CAD build for the part. Positions are in the model's coordinates, mm. Give positions to 0.01 mm unless a question says otherwise; leave off trailing zeros. Loops run counter-clockwise (first coordinate to the right, second up) from the corner with the lowest first, then second, coordinate; pieces in that order, holes last.
Autodesk Fusion 360 part; units mm, degrees
sketch "Sketch1" plane through (0, 0, 0) normal (0, 1, 0) x (1, 0, 0)
  line L0 (0.6394, 2.8043) -> (0.4754, 3.1598)
  line L1 (322.165, 133.829) -> (322.508, 133.638)
  line L2 (0.4754, 3.1598) -> (0.339, 3.5278)
  line L3 (324.895, 129.374) -> (324.896, 5.0726)
  line L4 (0.2329, 3.9067) -> (0.1557, 4.2912)
  line L5 (0.339, 3.5278) -> (0.2329, 3.9067)
  line L6 (0.831, 2.4612) -> (0.6394, 2.8043)
  line L7 (0.1557, 4.2912) -> (0.1102, 4.6812)
  line L8 (321.809, 0.4548) -> (321.441, 0.3183)
  line L9 (320.678, 0.135) -> (320.288, 0.0896)
  line L10 (1.2912, 1.8259) -> (1.0487, 2.1346)
  line L11 (324.879, 129.767) -> (324.895, 129.374)
  line L12 (324.514, 131.288) -> (324.651, 130.92)
  line L13 (323.698, 132.623) -> (323.941, 132.314)
  line L14 (324.159, 2.4612) -> (323.941, 2.1346)
  line L15 (324.651, 3.5278) -> (324.514, 3.1598)
  line L16 (323.431, 1.5379) -> (323.143, 1.2705)
  line L17 (324.35, 2.8043) -> (324.159, 2.4612)
  line L18 (324.757, 130.542) -> (324.834, 130.157)
  line L19 (324.834, 4.2912) -> (324.757, 3.9067)
  line L20 (322.508, 0.8103) -> (322.165, 0.6187)
  line L21 (324.757, 3.9067) -> (324.651, 3.5278)
  line L22 (323.698, 1.8259) -> (323.431, 1.5379)
  line L23 (322.834, 1.028) -> (322.508, 0.8103)
  line L24 (322.508, 133.638) -> (322.834, 133.42)
  line L25 (320.288, 0.0896) -> (319.896, 0.073)
  line L26 (322.834, 133.42) -> (323.143, 133.178)
  line L27 (321.062, 134.236) -> (321.441, 134.13)
  line L28 (323.143, 133.178) -> (323.431, 132.91)
  line L29 (324.651, 130.92) -> (324.757, 130.542)
  line L30 (3.9274, 0.2122) -> (3.5485, 0.3183)
  line L31 (324.35, 131.644) -> (324.514, 131.288)
  line L32 (320.288, 134.359) -> (320.678, 134.313)
  line L33 (320.678, 134.313) -> (321.062, 134.236)
  line L34 (321.441, 134.13) -> (321.809, 133.993)
  line L35 (323.941, 132.314) -> (324.159, 131.987)
  line L36 (321.062, 0.2122) -> (320.678, 0.135)
  line L37 (323.143, 1.2706) -> (322.834, 1.028)
  line L38 (321.441, 0.3183) -> (321.062, 0.2122)
  line L39 (319.896, 0.073) -> (5.0946, 0.073)
  line L40 (324.514, 3.1598) -> (324.35, 2.8043)
  line L41 (324.896, 5.0726) -> (324.879, 4.6812)
  line L42 (324.834, 130.157) -> (324.879, 129.767)
  line L43 (5.0946, 0.073) -> (4.7019, 0.0896)
  line L44 (324.879, 4.6812) -> (324.834, 4.2912)
  line L45 (321.809, 133.993) -> (322.165, 133.829)
  line L46 (3.1805, 0.4548) -> (2.825, 0.6187)
  line L47 (319.896, 134.374) -> (320.288, 134.359)
  line L48 (4.3119, 0.135) -> (3.9274, 0.2122)
  line L49 (2.1553, 1.028) -> (1.8466, 1.2706)
  line L50 (2.825, 0.6187) -> (2.4819, 0.8103)
  line L51 (2.4819, 0.8103) -> (2.1553, 1.028)
  line L52 (324.159, 131.987) -> (324.35, 131.644)
  line L53 (322.165, 0.6187) -> (321.809, 0.4548)
  line L54 (4.7019, 0.0896) -> (4.3119, 0.135)
  line L55 (3.5485, 0.3183) -> (3.1805, 0.4548)
  line L56 (323.941, 2.1346) -> (323.698, 1.8259)
  line L57 (323.431, 132.91) -> (323.698, 132.623)
  line L58 (3.1805, 133.993) -> (3.5485, 134.13)
  line L59 (1.8466, 133.178) -> (2.1553, 133.42)
  line L60 (4.3119, 134.313) -> (4.7019, 134.359)
  line L61 (4.7019, 134.359) -> (5.0946, 134.375)
  line L62 (5.0946, 134.375) -> (319.896, 134.374)
  line L63 (3.5485, 134.13) -> (3.9274, 134.236)
  line L64 (1.5586, 1.5379) -> (1.2912, 1.8259)
  line L65 (0.6394, 131.644) -> (0.831, 131.987)
  line L66 (0.4754, 131.288) -> (0.6394, 131.644)
  line L67 (0.1102, 129.767) -> (0.1557, 130.157)
  line L68 (2.1553, 133.42) -> (2.4819, 133.638)
  line L69 (1.8466, 1.2706) -> (1.5586, 1.5379)
  line L70 (0.1102, 4.6812) -> (0.0937, 5.0739)
  line L71 (314.895, 124.375) -> (314.895, 10.0748)
  line L72 (10.0941, 124.375) -> (314.895, 124.375)
  line L73 (3.9274, 134.236) -> (4.3119, 134.313)
  line L74 (0.831, 131.987) -> (1.0487, 132.314)
  line L75 (1.0487, 132.314) -> (1.2912, 132.623)
  line L76 (314.895, 10.0748) -> (10.0941, 10.0748)
  line L77 (0.2329, 130.542) -> (0.339, 130.92)
  line L78 (0.339, 130.92) -> (0.4754, 131.288)
  line L79 (0.0937, 5.0739) -> (0.0951, 129.374)
  line L80 (1.2912, 132.623) -> (1.5586, 132.91)
  line L81 (0.1557, 130.157) -> (0.2329, 130.542)
  line L82 (2.825, 133.829) -> (3.1805, 133.993)
  line L83 (0.0951, 129.374) -> (0.1102, 129.767)
  line L84 (10.0941, 10.0748) -> (10.0941, 124.375)
  line L85 (1.5586, 132.91) -> (1.8466, 133.178)
  line L86 (2.4819, 133.638) -> (2.825, 133.829)
  line L87 (1.0487, 2.1346) -> (0.831, 2.4612)
extrude "Extrude1" add sketch "Sketch1" along normal blind 3
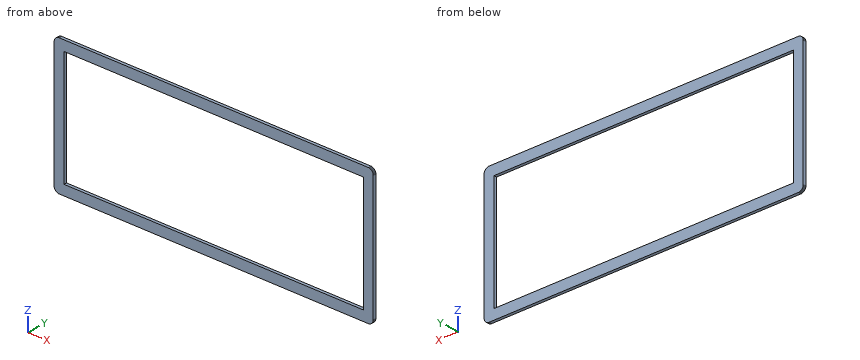
1. Saw through at A-A, the plane x = 276. List the corners of the cut face in (y, z) (3 decimals).
Responses:
outline: (0, -134.374) - (3, -134.374) - (3, -124.375) - (0, -124.375) - close; (0, -10.075) - (3, -10.075) - (3, -0.073) - (0, -0.073) - close
2. Saw through at B-B, the plane z = -26.5. List the corners of the cut face in (x, y) (3 decimals), and give its area (3 significant figures).
Responses:
outline: (0.094, 0) - (10.094, 0) - (10.094, 3) - (0.094, 3) - close; (314.895, 0) - (324.896, 0) - (324.896, 3) - (314.895, 3) - close
area: 60.0 mm2
3. Probe line 1 along X through (y, z) = (0.85, -64.5) (3 decimals); line 2 along Z through (x, y) = (66, 0.45) (3 decimals); line 3 along X through (y, z) = (2.8, -126.5). List the from-to ranges inside material, lowest first.
Responses:
line 1: x = 0.094 to 10.094, 314.895 to 324.896
line 2: z = -134.375 to -124.375, -10.075 to -0.073
line 3: x = 0.1 to 324.9
